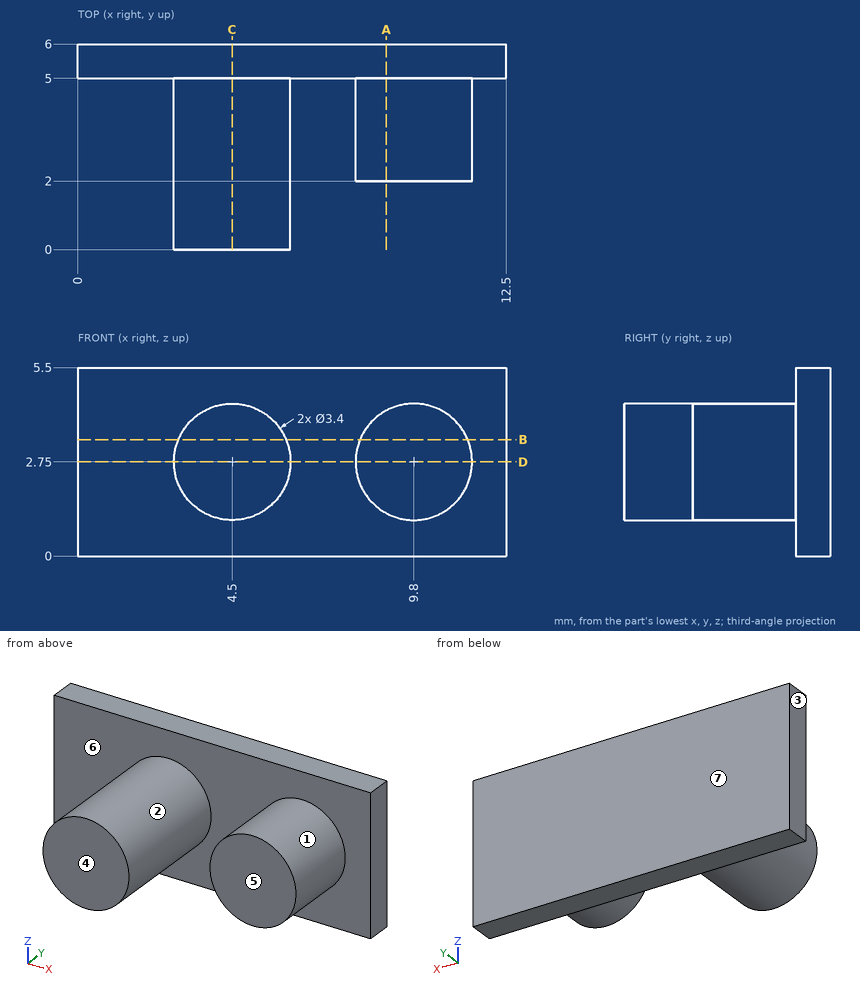
Input: dimensioned drawing with shaded views. Units: mm. Origin: part minimum x, y, z. A direction names the side the tool comes from. Give positions to 0.01 mm unless a question says otherwise; leave off trailing zeros. Write each loop counter-clockwise with the first axis right and the second up, starting at its lowest first coordinate (ties: lowest second). Pieces come first, ordered by that corner, then holes. Notation, with made-up numbers: (-2, -20.5) - (13, -20.5) arc R27 cw to (13, -2.5) - close; hole circle Ø8 at (12.5, -2.5). An arc over 180 degrees is marked (long way). One line per item, written item: value. Start each with the question number.
Q1. Section query A-A, the plane x = 9. Return the cut outline in (y, z), then the cut area to 3 significant figures.
Q2. Material intervals for probe 1 along X at (y, z) = (2.1, 2.7); probe 2 along Y at (x, z) = (1.25, 4.1); probe 3 along X at (y, z) = (4.65, 3.75), sorted ascending. Write a range as from..to.
Q3. First-contact query: pin 1 Ø1.5 at (x, y) = (3.5, 3) entering from -Z; pin 2 Ø2.5 at (x, z) = (9.5, 3.5) entering from -Y; pin 3 Ø1.5 at (x, y) = (6.5, 3.5) entering from -Z. Flat tips, straight axial feed; report the tip coordinate or a pass-through.
Q4. Set-up query: the marked faces 5, 6 and 7. Return all of +Z, -Z, +X, -X, +Y, -Y with unobstructed straight access to the full face (end or side cutting, diameter ignored); none if empty.
Q5. Section query C-C, the plane x = 4.5. Return the cut outline in (y, z).
Q6. Section query B-B, the plane z = 3.4. Return the cut outline in (x, y).
Q7. Section query D-D, the plane z = 2.75. Return the cut outline in (x, y), then the cut area to 3 significant figures.
Q8. Draft query along X for the marked faces 1, 2, 3 and 4. Return one class per face: +X half, -X half, draft (parallel to the pull), parting line (faces both ways), or undercut.
Answer:
1. outline: (2, 1.25) - (5, 1.25) - (5, 0) - (6, 0) - (6, 5.5) - (5, 5.5) - (5, 4.25) - (2, 4.25) - close
1. area: 14.5 mm2
2. probe 1: x = 2.8..6.2, 8.1..11.5
2. probe 2: y = 5..6
2. probe 3: x = 3.13..5.87, 8.43..11.17
3. pin 1: stops at z = 1.07
3. pin 2: stops at y = 2
3. pin 3: stops at z = 1.6
4. face 5: +Z, -Z, +X, -Y
4. face 6: -Y
4. face 7: +Z, -Z, +X, -X, +Y
5. outline: (0, 1.05) - (5, 1.05) - (5, 0) - (6, 0) - (6, 5.5) - (5, 5.5) - (5, 4.45) - (0, 4.45) - close
6. outline: (0, 5) - (2.93, 5) - (2.93, 0) - (6.07, 0) - (6.07, 5) - (8.23, 5) - (8.23, 2) - (11.37, 2) - (11.37, 5) - (12.5, 5) - (12.5, 6) - (0, 6) - close
7. outline: (0, 5) - (2.8, 5) - (2.8, 0) - (6.2, 0) - (6.2, 5) - (8.1, 5) - (8.1, 2) - (11.5, 2) - (11.5, 5) - (12.5, 5) - (12.5, 6) - (0, 6) - close
7. area: 39.7 mm2
8. face 1: undercut
8. face 2: undercut
8. face 3: -X half
8. face 4: draft
